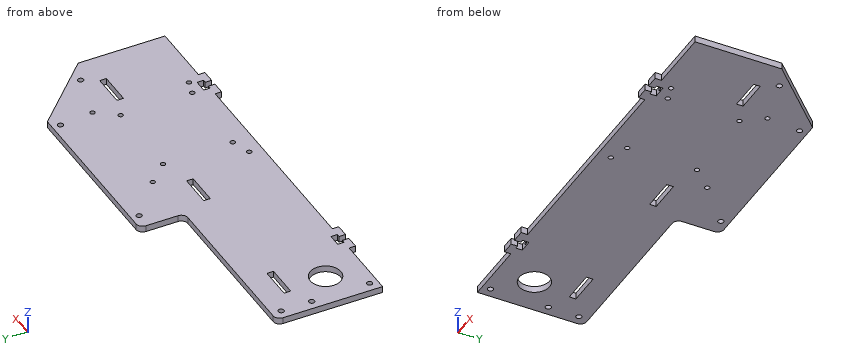
from build123d import *

# Parameters (mm, degrees)
SKETCH_1_R             = 9.5
SKETCH_1_R_2           = 1.5
SKETCH_1_W             = 20.5
SKETCH_1_H             = 4.1
SM_BASE_FLANGE_1_DEPTH = 4
SKETCH_6_R             = 1.75
CUT_EXTRUDE_1_DEPTH    = 267.640207021
SKETCH_8_R             = 1
SKETCH_8_R_2           = 0.822154456
CUT_EXTRUDE_3_DEPTH    = 10


# Sheet-metal steps are written as plain solids
with BuildPart() as part:
    # Sketch 1 → Базовая кромка1 (new body)
    with BuildSketch(Plane.XY):
        with BuildLine():
            Line((52, -59), (60, -59))
            Line((60, -59), (60, -55))
            Line((60, -55), (200, -55))
            Line((200, -55), (200, -59))
            Line((200, -59), (208, -59))
            Line((208, -59), (208, -55))
            Line((208, -55), (206, -55))
            Line((206, -55), (206, -51))
            Line((206, -51), (214, -51))
            Line((214, -51), (214, -55))
            Line((214, -55), (212, -55))
            Line((212, -55), (212, -59))
            Line((212, -59), (220, -59))
            Line((220, -59), (220, -55))
            Line((220, -55), (260, -55))
            Line((260, -55), (260, -1))
            Line((260, -1), (220, 39))
            Line((220, 39), (120, 39))
            Line((120, 39), (114, 39))
            ThreePointArc((114, 39), (111.171572875, 37.828427125), (110, 35))
            Line((110, 35), (110, 15))
            ThreePointArc((110, 15), (108.828427125, 12.171572875), (106, 11))
            Line((106, 11), (4, 11))
            ThreePointArc((4, 11), (1.171572875, 9.828427125), (0, 7))
            Line((0, 7), (0, 0))
            Line((0, 0), (0, -55))
            Line((0, -55), (40, -55))
            Line((40, -55), (40, -59))
            Line((40, -59), (48, -59))
            Line((48, -59), (48, -55))
            Line((48, -55), (46, -55))
            Line((46, -55), (46, -51))
            Line((46, -51), (54, -51))
            Line((54, -51), (54, -55))
            Line((54, -55), (52, -55))
            Line((52, -55), (52, -59))
        make_face()
        with Locations((23, -31.5)):
            Circle(SKETCH_1_R, mode=Mode.SUBTRACT)
        with Locations((156, -43)):
            Circle(SKETCH_1_R_2, mode=Mode.SUBTRACT)
        with Locations((206.7, 0.4)):
            Circle(SKETCH_1_R_2, mode=Mode.SUBTRACT)
        with Locations((156, 0.4)):
            Circle(SKETCH_1_R_2, mode=Mode.SUBTRACT)
        with Locations((206.7, -44.2)):
            Circle(SKETCH_1_R_2, mode=Mode.SUBTRACT)
        with Locations((144, -47)):
            Circle(SKETCH_1_R_2, mode=Mode.SUBTRACT)
        with Locations((216, -47)):
            Circle(SKETCH_1_R_2, mode=Mode.SUBTRACT)
        with Locations((216, 13)):
            Circle(SKETCH_1_R_2, mode=Mode.SUBTRACT)
        with Locations((144, 13)):
            Circle(SKETCH_1_R_2, mode=Mode.SUBTRACT)
        with Locations((30, -6.05)):
            Rectangle(SKETCH_1_W, SKETCH_1_H, mode=Mode.SUBTRACT)
        with Locations((230, -6.169027082)):
            Rectangle(SKETCH_1_W, SKETCH_1_H, mode=Mode.SUBTRACT)
        with Locations((126, -6.05)):
            Rectangle(SKETCH_1_W, SKETCH_1_H, mode=Mode.SUBTRACT)
    extrude(amount=-SM_BASE_FLANGE_1_DEPTH)

    # Эскиз6 → Вырез-Вытянуть1 (cut, through all)
    with BuildSketch(Plane.XY):
        with Locations((6, 5)):
            Circle(SKETCH_6_R)
        with Locations((120, 34)):
            Circle(SKETCH_6_R)
        with Locations((214, 34)):
            Circle(SKETCH_6_R)
        with Locations((245.514718626, 5)):
            Circle(SKETCH_6_R)
        with Locations((6, -14)):
            Circle(SKETCH_6_R)
        with Locations((6, -50)):
            Circle(SKETCH_6_R)
    extrude(amount=-CUT_EXTRUDE_1_DEPTH, mode=Mode.SUBTRACT)

    # Эскиз8 → Вырез-Вытянуть3 (cut)
    with BuildSketch(Plane.XZ.offset(55)):
        with Locations((210, -2)):
            Circle(SKETCH_8_R)
        with Locations((50, -2)):
            Circle(SKETCH_8_R_2)
    extrude(amount=-CUT_EXTRUDE_3_DEPTH, mode=Mode.SUBTRACT)


solid = part.part
Read the model definition and answer for the solid it produces. Units are mm, in the model's axes. Coordinates: 2 decimals unless noted, no trailing zeros. Write each loop counter-clockwise with the first axis right and the second up, starting at its lowest first coordinate (ties: lowest second). Pieces come first, ordered by that corner, then holes. Notation, with made-up numbers: M 11.5,75.5 L 44.5,75.5 A26 ccw 44.5,106.5 Z; hole C 26.25,-31 d10. An arc over 180 degrees is marked long. Use a Markdown table: item, result.
Q1. The part is cut by section B-B, the plane x = 90.5. Write down the section's boundary in (y, z).
Answer block:
| item | result |
|---|---|
| outline | M -55,-4 L 11,-4 L 11,0 L -55,0 Z |
Q2. Each of these flat-tipped pins is pushed along its axis until it touches: pin 1 Ø1 at (x, z) = (210, -2) entering from -Y; pin 2 Ø1 at (x, z) = (53, -2) entering from +Y; pin 3 Ø12 at (x, y) = (225.5, 11) entering from +Z. Where does it stop, or does it pass through?
Answer block:
| item | result |
|---|---|
| pin 1 | stops at y = -45 |
| pin 2 | stops at y = 11 |
| pin 3 | stops at z = 0 |
Q3. Straight lines are drawn through the part: L1, parallel to Y at x = 206.7, z = -1.55; L2, parallel to Y at x = 156, z = -2.45; L3, parallel to X at y = -6, z = -3.75. For each, find the intervals that lie inside material, in ascending order. Write a range as [from, to].
Answer block:
| item | result |
|---|---|
| L1 | y = [-59, -55], [-51, -45.7], [-42.7, -1.1], [1.9, 39] |
| L2 | y = [-55, -44.5], [-41.5, -1.1], [1.9, 39] |
| L3 | x = [0, 19.75], [40.25, 115.75], [136.25, 219.75], [240.25, 260] |
Q4. The part is cut by section A-A, the plane x = 224. Write down the section's boundary in (y, z), then the cut area to 3 significant figures.
Answer block:
| item | result |
|---|---|
| outline | M -55,-4 L -8.22,-4 L -8.22,0 L -55,0 Z; M -4.12,-4 L 35,-4 L 35,0 L -4.12,0 Z |
| area | 344 mm2 |
